from build123d import *

# Parameters (mm, degrees)
F0_W     = 58.2168
F0_H     = 22.225
F1_DEPTH = 48.26
F3_DEPTH = 48.261
F5_DEPTH = 7.9502
F7_DEPTH = 14.2758


with BuildPart() as f1:
    # F0 (on Front) → F1 (new body)
    with BuildSketch(Plane.XZ):
        Rectangle(F0_W, F0_H)
    extrude(amount=F1_DEPTH)

    # F2 (on face) → F3 (cut, through all)
    with BuildSketch(Plane.XZ.offset(48.26)):
        Polygon((-22.2504, 11.1125), (-20.0112557785, 2.7559), (20.0112557785, 2.7559), (22.2504, 11.1125), (29.1084, 11.1125), (29.1084, 14.9114290252), (-29.1084, 14.9114290252), (-29.1084, 11.1125), align=None)
    extrude(amount=-F3_DEPTH, mode=Mode.SUBTRACT)

    # F4 (on face) → F5 (cut)
    with BuildSketch(Plane(origin=(0, 0, -11.1125), x_dir=(1, 0, 0), z_dir=(0, 0, -1))):
        with BuildLine():
            Line((8.509, 17.653), (8.509, 30.353))
            ThreePointArc((8.509, 30.353), (0, 38.862), (-8.509, 30.353))
            Line((-8.509, 30.353), (-8.509, 17.653))
            ThreePointArc((-8.509, 17.653), (0, 9.144), (8.509, 17.653))
        make_face()
    extrude(amount=-F5_DEPTH, mode=Mode.SUBTRACT)

    # F6 (on face) → F7 (cut, through all)
    with BuildSketch(Plane(origin=(0, 0, -3.1623), x_dir=(1, 0, 0), z_dir=(0, 0, -1))):
        with BuildLine():
            Line((-5.08, 30.353), (-5.08, 24.4791761624))
            ThreePointArc((-5.08, 24.4791761624), (0, 9.144), (5.08, 24.4791761624))
            Line((5.08, 24.4791761624), (5.08, 30.353))
            ThreePointArc((5.08, 30.353), (0, 35.433), (-5.08, 30.353))
        make_face()
    extrude(amount=-F7_DEPTH, mode=Mode.SUBTRACT)


solid = f1.part
Verification items for the finished model (mm, model axes). A direction names the side the tool comes from. Round coordinates to 2 decimals unless told otherwise and drop trailing zeros. Loops run counter-clockwise (first coordinate to the right, second up) from the corner with the lowest first, then second, coordinate; pieces in that order, holes last. Notation, with made-up numbers: (-4.75, -15.75) - (6.25, -15.75) arc R15 ccw to (6.25, 13.25) - close; hole circle Ø8 at (37, -1). An arc over 180 degrees is marked (long way). Answer in a Markdown table with one row per item. Add a question column.
Q1. Tool access check on faces 4 (the face through (-9, -24, 2.756)), 5 (the face through (-13, -24, -11.112)), 6 (the face through (-5.08, -27, 0)), 7 (the face through (-2, -35.5, -3.162)), 8 (the face through (29.108, -24, 0)). Record the directions out of +Z, -Z, +X, -X, +Y, -Y that give a thin tool (end or side, any length) a straight path to the whole face; none if there is none.
Q2. Release check for a two-part mould opening along Y. For faces 1 (the face through (0.19, -38.86, -7.19)), 2 (the face through (0, 0, -2)), 3 (the face through (-29.108, -24, 0)) record: pulls with the +Y half, pulls with the -Y half, needs draft (parallel to the pull), parting line crosses it, or undercut.
Q3. Section check A-A on x = 0. Enter the section's corners in (y, z), plus the area to 3 significant figures.
Q4. Section check D-D on z = 7. Enter the section's corners in (x, y).
Q5. Section check B-B on z = -8.25. Enter the section's corners in (x, y).
Q6. Section check C-C on y = -45. Enter the section's corners in (x, z).
Q7. Material ranges on line 1 (X direction, y = -27, z = -6); line 2 (Y direction, x = 0, z = -0.25); line 3 (Y direction, x = 0, z = -4), recorded low to high.
Q8. Gauge pin test, flat ends, axial feed: pin 1 (19.5 mm diameter, centred on x = 0, y = -17.653, fed in from +Z); pin 2 (5 mm diameter, centred on x = -2.5, y = -27, fed in from -Z). Record the tip position at first contact, or that the pin passes through.
Found:
| question | item | result |
|---|---|---|
| 1 | face 4 | +Z, +Y, -Y |
| 1 | face 5 | -Z, +X, -X, +Y, -Y |
| 1 | face 6 | +Z, -Z |
| 1 | face 7 | -Z |
| 1 | face 8 | +Z, -Z, +X, +Y, -Y |
| 2 | face 1 | undercut |
| 2 | face 2 | pulls with the +Y half |
| 2 | face 3 | needs draft |
| 3 | outline | (-48.26, -11.11) - (-38.86, -11.11) - (-38.86, -3.16) - (-35.43, -3.16) - (-35.43, 2.76) - (-48.26, 2.76) - close; (-9.14, -11.11) - (0, -11.11) - (0, 2.76) - (-9.14, 2.76) - close |
| 3 | area | 277 mm² |
| 4 | outline | (-29.11, -48.26) - (-21.15, -48.26) - (-21.15, 0) - (-29.11, 0) - close; (21.15, -48.26) - (29.11, -48.26) - (29.11, 0) - (21.15, 0) - close |
| 5 | outline | (-29.11, -48.26) - (29.11, -48.26) - (29.11, 0) - (-29.11, 0) - close; hole (-8.51, -30.35) arc R8.51 ccw to (8.51, -30.35) - (8.51, -17.65) arc R8.51 ccw to (-8.51, -17.65) - close |
| 6 | outline | (-29.11, -11.11) - (29.11, -11.11) - (29.11, 11.11) - (22.25, 11.11) - (20.01, 2.76) - (-20.01, 2.76) - (-22.25, 11.11) - (-29.11, 11.11) - close |
| 7 | line 1 | x = -29.11 to -8.51, 8.51 to 29.11 |
| 7 | line 2 | y = -48.26 to -35.43, -9.14 to 0 |
| 7 | line 3 | y = -48.26 to -38.86, -9.14 to 0 |
| 8 | pin 1 | stops at z = 2.76 |
| 8 | pin 2 | passes through |
